Could you check a few things on this drawing? It's one solid part, dimensions in mm from its lowest x, y, z. Coordinates: 2 decimals unless noted, no trailing zeros. Order: outer loops, then holes, each group sorted by start corner. A loop starts at its lowest first (then second) coordinate and runs counter-clockwise, first axis right, second up. Notation, with made-up numbers: (-13.5, 26.25) - (19.5, 26.25) arc R23 cw to (19.5, 41.25) - close; hole circle Ø11 at (59.25, 12.5). An arc over 180 degrees is marked (long way). Return JSON: item names as keys, results as strings. Group by question number.
1) Imagine slicing it at A-A (x = 0.85). Write out the boundary of the cut face in (y, z).
2) If I drill on line 1 along Y through (x, z) = (1.6, 4.5), over which ranges is the centre line in solid material (lowest first)?
3) For pin 1 Ø0.9 at (x, z) = (2, 26.5) entering from +Y; pin 2 Ø1.5 at (x, y) = (2, 138) entering from +Z, each with a flat end and sliding along its axis, tell me the tip position at first contact or that it passes through.
4) Imagine slicing it at B-B (z = 22.5). Write out the boundary of the cut face in (x, y).
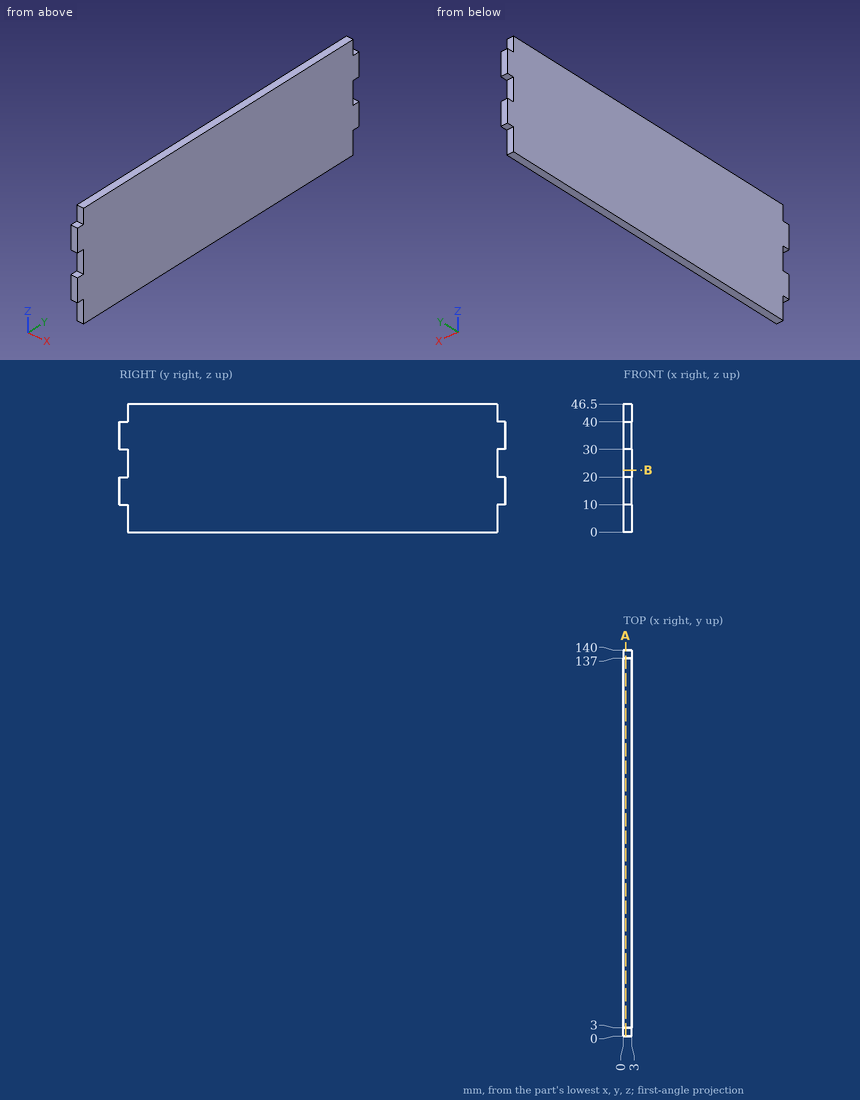
Calculated:
{
 "1": {"outline": "(0, 10) - (3, 10) - (3, 0) - (137, 0) - (137, 10) - (140, 10) - (140, 20) - (137, 20) - (137, 30) - (140, 30) - (140, 40) - (137, 40) - (137, 46.5) - (3, 46.5) - (3, 40) - (0, 40) - (0, 30) - (3, 30) - (3, 20) - (0, 20) - close"},
 "2": {"line 1": "3 to 137"},
 "3": {"pin 1": "y = 137", "pin 2": "z = 40"},
 "4": {"outline": "(0, 3) - (3, 3) - (3, 137) - (0, 137) - close"}
}
